Design review of the part built by this model. Coordinates are the model's own, in mm. A direction names the side the tool comes from. Round coordinates to 2 decimals unless told otherwise and drop trailing zeros. Loops run counter-clockwise (first coordinate to the right, second up) from the corner with the lowest first, then second, coordinate; pieces in that order, holes last. Notation, with made-up numbers: (-16.75, 60.25) - (-12.75, 60.25) arc R11 cw to (-12.75, 71.25) - close; hole circle Ø2 at (37.5, 63.25). An arc over 180 degrees is marked (long way). Use one line per item in the form item = value. Start each with the question number.
(1) We need section A-A, the plane y = -9. Write out the cut boundary in (x, z).
(2) We need section C-C, the plane x = -7. Write out the cut boundary in (y, z).
(3) Machinability: for faces 1 (the flat face through (76.2, -32, 2)), 2 (the cylindrical face through (-29.84, -122.46, 2.41)), 3 (the flat face through (44.45, -149, 2)), which of the approach directions +Z, -Z, +X, -X, +Y, -Y give a long, thin tool a straight path to every point of the face, cutting with its end or side? Answer none if there is none.
(4) The part is to be moulded in two halves that separate along X. For faces 4 (the flat face through (-1, -55, 0)), 5 (the cylindrical face through (29.94, -122.56, 2.41)), 6 (the cylindrical face through (-42.64, -163.19, 2.41)), 7 (the cylindrical face through (-73.87, -78.58, 2.41)), say which applies: released by +X, released by -X, zero draft, split by the parting line, or undercut.
(5) For pin 1 (1.5 mm diameter, centred on x = 72.5, z = 0.5, fed in from +Y); pin 2 (0.7 mm diameter, centred on y = 6.5, z = 1.5, fed in from -X) (3 decimals); pin 3 (7.5 mm diameter, centred on x = 92.5, y = 6, fed in from +Z); pin 4 (3 mm diameter, centred on x = 18.5, y = -114.3, fed in from -Z), all flat-tipped, find the tip position at first contact; note any pin that passes through.
(6) We need section D-D, the plane z = 1.2. Give the number of separate pieces and of enclosed holes in the cut face, then the cut area to 3 significant figures.
(7) Wall thickness on probe 1 along X at (y, z) = (-55.5, 1.1); probe 2 along X at (y, z) = (-77.3, 2.1); probe 3 along X at (y, z) = (-146, 1.05): over which ranges is each line inside the solid? List them lowest first. Write a range as [from, to].
(8) We need section B-B, the plane x = 18.5. Write out the cut boundary in (y, z).
Autodesk Inventor part; units mm, degrees
ref_plane "YZ Plane" through (0, 0, 0) normal (1, 0, 0) x (0, 1, 0)
ref_plane "XZ Plane" through (0, 0, 0) normal (0, 1, 0) x (-1, 0, 0)
ref_plane "XY Plane" through (0, 0, 0) normal (0, 0, 1) x (1, 0, 0)
sketch "Sketch1" plane through (0, 0, 0) normal (0, 0, 1) x (1, 0, 0)
  line L0 (-133.35, 0) -> (133.35, 0)
  line L1 (0, -231.14) -> (0, 231.14)
  line L2 (-44.45, -165.1) -> (44.45, 165.1) construction
  line L3 (44.45, -165.1) -> (-44.45, 165.1) construction
  line L4 (-95.25, -88.9) -> (-44.45, -88.9)
  line L5 (-44.45, 88.9) -> (-95.25, 88.9)
  line L6 (-95.25, 88.9) -> (-95.25, -88.9)
  line L7 (-95.25, -88.9) -> (-44.45, 88.9) construction
  line L8 (-44.45, -88.9) -> (-95.25, 88.9) construction
  line L9 (95.25, -88.9) -> (44.45, -88.9)
  line L10 (44.45, 88.9) -> (95.25, 88.9)
  line L11 (95.25, 88.9) -> (95.25, -88.9)
  line L12 (95.25, -88.9) -> (44.45, 88.9) construction
  line L13 (44.45, -88.9) -> (95.25, 88.9) construction
  line L14 (44.45, -165.1) -> (44.45, -88.9)
  line L15 (44.45, 88.9) -> (44.45, 165.1)
  line L16 (-44.45, 165.1) -> (-44.45, 88.9)
  line L17 (-44.45, -88.9) -> (-44.45, -165.1)
  line L18 (-31.75, 120.65) -> (31.75, 120.65)
  line L19 (31.75, 120.65) -> (31.75, 165.1)
  line L20 (-31.75, 165.1) -> (-31.75, 120.65)
  line L21 (-31.75, 120.65) -> (31.75, 165.1) construction
  line L22 (31.75, 120.65) -> (-31.75, 165.1) construction
  line L23 (-31.75, -120.65) -> (31.75, -120.65)
  line L24 (31.75, -120.65) -> (31.75, -165.1)
  line L25 (-31.75, -165.1) -> (-31.75, -120.65)
  line L26 (-31.75, -120.65) -> (31.75, -165.1) construction
  line L27 (31.75, -120.65) -> (-31.75, -165.1) construction
  line L28 (44.45, 165.1) -> (31.75, 165.1)
  line L29 (-31.75, 165.1) -> (-44.45, 165.1)
  line L30 (-44.45, -165.1) -> (-31.75, -165.1)
  line L31 (31.75, -165.1) -> (44.45, -165.1)
  point P0 (0, 0)
  point P1 (-69.85, 0)
  point P2 (69.85, 0)
  point P3 (0, 142.875)
  point P4 (0, -142.875)
  dimension "d0" = 88.9
  dimension "d1" = 330.2
  dimension "d3" = 50.8
  dimension "d4" = 12.7
  dimension "d5" = 44.45
  dimension "d27" = 76.2
extrude "Extrusion1" add sketch "Sketch1" along normal blind 4.7625
sketch "Sketch2" plane through (0, 0, 4.7625) normal (0, 0, 1) x (1, 0, 0)
  line L0 (0, -231.14) -> (0, 231.14)
  line L1 (-133.35, 0) -> (133.35, 0)
  line L2 (31.75, -165.1) -> (44.45, -165.1)
  line L3 (44.45, -165.1) -> (44.45, -88.9)
  line L4 (-31.75, -120.65) -> (31.75, -120.65)
  point P0 (0, 0)
  point P1 (38.1, -158.75)
  point P2 (-38.1, -158.75)
  point P3 (38.1, 158.75)
  point P4 (-38.1, 158.75)
  point P5 (18.5, -114.3)
  point P6 (-18.5, -114.3)
  point P7 (-18.5, -77.3)
  point P8 (18.5, -77.3)
  point P9 (18.5, 77.3)
  point P10 (-18.5, 77.3)
  point P11 (18.5, 114.3)
  point P12 (-18.5, 114.3)
  dimension "d10" = 6.35
  dimension "d11" = 6.35
  dimension "d12" = 37
  dimension "d13" = 37
  dimension "d14" = 6.35
hole "Hole1" at (38.1, -158.75, 4.7625) at (-38.1, -158.75, 4.7625) at (38.1, 158.75, 4.7625) at (-38.1, 158.75, 4.7625) at (18.5, -114.3, 4.7625) at (-18.5, -114.3, 4.7625) at (-18.5, -77.3, 4.7625) at (18.5, -77.3, 4.7625) at (18.5, 77.3, 4.7625) at (-18.5, 77.3, 4.7625) at (18.5, 114.3, 4.7625) at (-18.5, 114.3, 4.7625) direction (0, 0, -1) diameter 4.7625 end through all
sketch "Sketch3" plane through (0, 0, 4.7625) normal (0, 0, 1) x (1, 0, 0)
  line L0 (73.8188, -76.2) -> (73.8187, 76.2) construction
  line L1 (76.2, -76.2) -> (76.2, 76.2)
  line L2 (71.4375, 76.2) -> (71.4375, -76.2)
  arc A0 (71.4375, -76.2) -> (76.2, -76.2) centre (73.8188, -76.2) ccw
  arc A1 (76.2, 76.2) -> (71.4375, 76.2) centre (73.8187, 76.2) ccw
  line L3 (-73.8188, -76.2) -> (-73.8188, 76.2) construction
  line L4 (-71.4375, -76.2) -> (-71.4375, 76.2)
  line L5 (-76.2, 76.2) -> (-76.2, -76.2)
  arc A2 (-76.2, -76.2) -> (-71.4375, -76.2) centre (-73.8188, -76.2) ccw
  arc A3 (-71.4375, 76.2) -> (-76.2, 76.2) centre (-73.8188, 76.2) ccw
  line L6 (0, -231.14) -> (0, 231.14)
  line L7 (-133.35, 0) -> (133.35, 0)
  line L8 (95.25, -88.9) -> (95.25, 88.9)
  point P0 (0, 0)
  point P1 (73.8187, 0)
  point P2 (-73.8187, 0)
  dimension "d22" = 152.4
  dimension "d23" = 4.7625
  dimension "d24" = 19.05
extrude "Extrusion2" cut sketch "Sketch3" along normal through all both and the other way through all
fillet "Fillet1" radius 6.35 16 edges at (44.45, 165.1, 2.3813) (31.75, 165.1, 2.3813) (95.25, 88.9, 2.3813) (31.75, 120.65, 2.3813) (-31.75, 120.65, 2.3813) (-31.75, 165.1, 2.3813) (-44.45, 165.1, 2.3813) (-95.25, 88.9, 2.3813) (-95.25, -88.9, 2.3813) (-44.45, -165.1, 2.3813) (-31.75, -165.1, 2.3813) (-31.75, -120.65, 2.3813) (31.75, -120.65, 2.3813) (31.75, -165.1, 2.3813) (44.45, -165.1, 2.3813) (95.25, -88.9, 2.3813)
fillet "Fillet2" radius 50.8 4 edges at (44.45, -88.9, 2.3813) (-44.45, -88.9, 2.3813) (-44.45, 88.9, 2.3813) (44.45, 88.9, 2.3813)
sketch "Sketch4" plane through (0, 0, 4.7625) normal (0, 0, 1) x (1, 0, 0)
  line L0 (-133.35, 0) -> (133.35, 0)
  line L1 (0, -231.14) -> (0, 231.14)
  line L2 (95.25, -82.55) -> (95.25, 82.55)
  line L3 (95.25, 12.7) -> (-95.25, 12.7)
  line L4 (-95.25, 12.7) -> (-95.25, 165.1)
  line L5 (-95.25, 165.1) -> (95.25, 165.1)
  line L6 (95.25, 165.1) -> (95.25, 12.7)
  arc A0 (-31.75, 158.75) -> (-44.45, 158.75) centre (-38.1, 158.75) ccw
  point P0 (0, 0)
  point P1 (-95.25, 82.55)
  dimension "d30" = 12.7
extrude "Extrusion3" cut sketch "Sketch4" along normal through all both and the other way through all contours L3 L4 L5 L1 | L1 L5 L6 L2 L3
sketch "Sketch5" plane through (0, 0, 4.7625) normal (0, 0, 1) x (1, 0, 0)
  line L0 (-95.25, 12.7) -> (-76.2, 12.7)
  line L1 (-76.2, 12.7) -> (-85.725, 12.7)
  line L2 (-85.725, 12.7) -> (-85.725, 0)
  line L3 (-85.725, 0) -> (-76.2, 0)
  line L4 (-76.2, 0) -> (-76.2, 12.7)
  line L5 (71.4375, 12.7) -> (-71.4375, 12.7)
  line L6 (0, 0) -> (-35.7188, 0)
  line L7 (-35.7188, 0) -> (-35.7187, 12.7)
  line L8 (-35.7187, 12.7) -> (0, 12.7)
  line L9 (0, 12.7) -> (0, 0)
  line L10 (71.4375, 12.7) -> (35.7188, 12.7)
  line L11 (35.7188, 12.7) -> (35.7188, 0)
  line L12 (35.7188, 0) -> (71.4375, 0)
  line L13 (71.4375, 0) -> (71.4375, 12.7)
  line L14 (95.25, -82.55) -> (95.25, 12.7)
  line L15 (95.25, 12.7) -> (85.725, 12.7)
  line L16 (85.725, 12.7) -> (85.725, 0)
  line L17 (85.725, 0) -> (95.25, 0)
  line L18 (95.25, 0) -> (95.25, 12.7)
  line L19 (95.25, 12.7) -> (76.2, 12.7)
  point P0 (-85.725, 12.7)
  dimension "d33" = 35.7188
  dimension "d34" = 35.7188
extrude "Extrusion4" cut sketch "Sketch5" against normal blind 2.3813
sketch "Sketch6" plane through (0, 0, 0) normal (0, 0, -1) x (-1, 0, 0)
  line L0 (95.25, 12.7) -> (95.25, -82.55)
  line L1 (85.725, 0) -> (95.25, 0)
  line L2 (95.25, 0) -> (95.25, 12.7)
  line L3 (95.25, 12.7) -> (85.725, 12.7)
  line L4 (85.725, 12.7) -> (85.725, 0)
  line L5 (71.4375, 12.7) -> (-71.4375, 12.7)
  line L6 (35.7188, 0) -> (71.4375, 0)
  line L7 (71.4375, 0) -> (71.4375, 12.7)
  line L8 (71.4375, 12.7) -> (35.7188, 12.7)
  line L9 (35.7188, 12.7) -> (35.7188, 0)
  line L10 (0, 0) -> (35.7188, 0)
  line L11 (0, 0) -> (-35.7188, 0)
  line L12 (-35.7188, 0) -> (-35.7188, 12.7)
  line L13 (-35.7188, 12.7) -> (0, 12.7)
  line L14 (0, 12.7) -> (0, 0)
  line L15 (-85.725, 0) -> (-85.725, 12.7)
  line L16 (-76.2, 12.7) -> (-76.2, -76.2)
  line L17 (-85.725, 0) -> (-76.2, 0)
  line L18 (-76.2, 0) -> (-76.2, 12.7)
  line L19 (-76.2, 12.7) -> (-85.725, 12.7)
  line L20 (-85.725, 12.7) -> (-85.725, 0)
extrude "Extrusion5" cut sketch "Sketch6" against normal blind 2.3813 contours L0 L1 L4 L3 | L7 L6 L9 L5 | L14 L11 L12 L5 | L15 L19 L16 L17
sketch "Sketch7" plane through (0, 0, 0) normal (0, 0, -1) x (-1, 0, 0)
  line L0 (71.4375, 12.7) -> (71.4375, 0)
  line L1 (0, -200.66) -> (0, 48.26)
  line L2 (-35.7188, 12.7) -> (-71.4375, 12.7)
  line L3 (-85.725, 0) -> (-85.725, 12.7)
  point P0 (0, 0)
  point P1 (80.9625, 6.35)
  point P2 (65.0875, 6.35)
  point P3 (-80.9625, 6.35)
  point P4 (-65.0875, 6.35)
  dimension "d39" = 6.35
  dimension "d40" = 6.35
  dimension "d41" = 4.7625
hole "Hole2" at (-80.9625, 6.35, 0) at (-65.0875, 6.35, 0) at (80.9625, 6.35, 0) at (65.0875, 6.35, 0) direction (0, 0, 1) diameter 4.7625 end through all
properties part number "RC_CAR_BASE_PLATE"
Data:
q1.outline = (-95.25, 0) - (-76.2, 0) - (-76.2, 4.76) - (-95.25, 4.76) - close; (-71.44, 0) - (71.44, 0) - (71.44, 4.76) - (-71.44, 4.76) - close; (76.2, 0) - (95.25, 0) - (95.25, 4.76) - (76.2, 4.76) - close
q2.outline = (-120.65, 0) - (12.7, 0) - (12.7, 2.38) - (0, 2.38) - (0, 4.76) - (-120.65, 4.76) - close
q3.face_1 = +Z, -Z, +Y
q3.face_2 = +Z, -Z, -Y
q3.face_3 = +Z, -Z, +X, -Y
q4.face_4 = zero draft
q4.face_5 = undercut
q4.face_6 = released by -X
q4.face_7 = undercut
q5.pin_1 = -77.38
q5.pin_2 = -85.725
q5.pin_3 = 2.38
q5.pin_4 = through
q6.separate_pieces = 1
q6.enclosed_holes = 8
q6.area = 22,200 mm^2
q7.probe_1 = [-95.25, -76.2], [-71.44, 71.44], [76.2, 95.25]
q7.probe_2 = [-95.25, -75.93], [-71.71, -20.88], [-16.12, 16.12], [20.88, 71.71], [75.93, 95.25]
q7.probe_3 = [-44.45, -31.75], [31.75, 44.45]
q8.outline = (-120.65, 0) - (-116.68, 0) - (-116.68, 4.76) - (-120.65, 4.76) - close; (-111.92, 0) - (-79.68, 0) - (-79.68, 4.76) - (-111.92, 4.76) - close; (-74.92, 0) - (0, 0) - (0, 2.38) - (12.7, 2.38) - (12.7, 4.76) - (-74.92, 4.76) - close
